Check sheet for the drawn part. Datum: minimum x, y, z corner. Units: mm. A direction names the side the tool comes from. Coordinates: 2 decimals unless noted, no trailing zeros. Write each loop counter-clockwise with the first axis right and the second up, starting at its lowest first coordinate (ties: lowest second). Pieces come first, ordered by that corner, then holes. Notation, with made-up numbers: (-9, -23.75) -> (12, -23.75) arc R24 cw to (12, -0.75) -> close; hole circle Ø4 at (37.5, -34). An arc over 180 degrees is marked (long way). One line per question, with ' | ' between items.
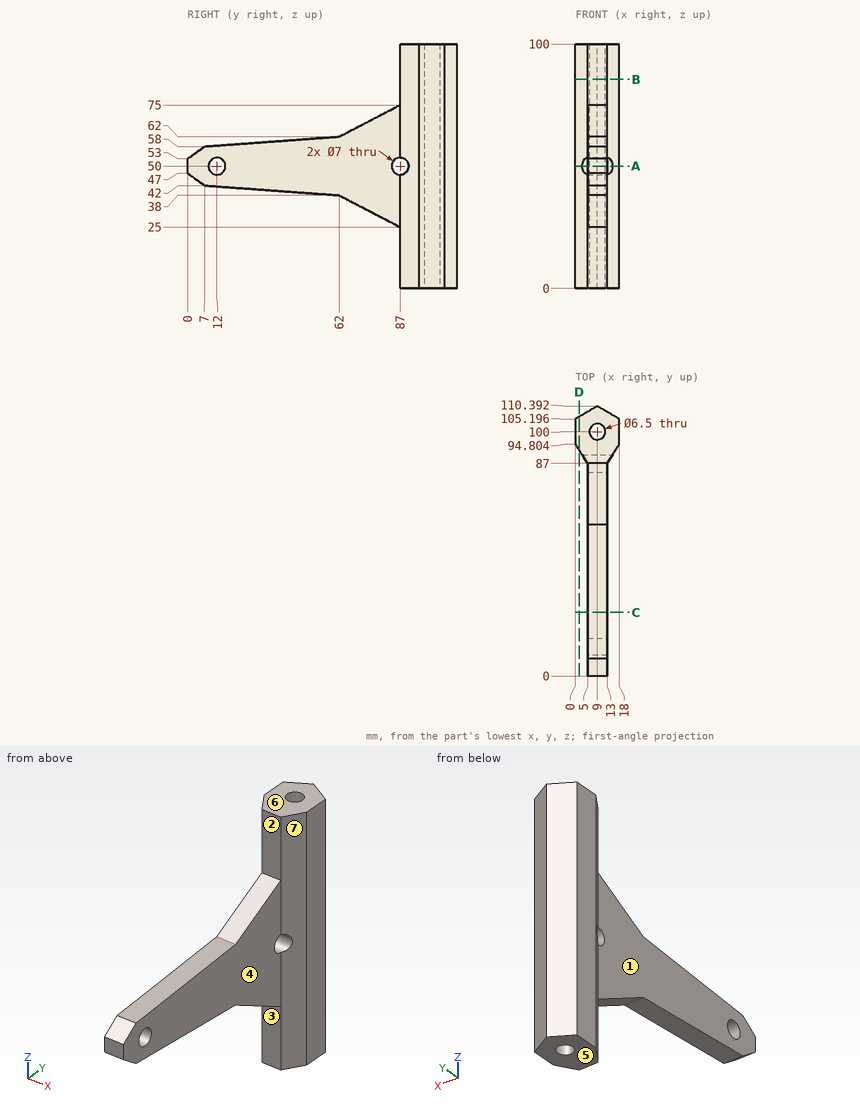
1. Tool access check on the marked faces 1, 2, 3 and 4. Record the directions out of +Z, -Z, +X, -X, +Y, -Y that give a thin tool (end or side, any length) a straight path to the whole face; none if there is none.
Worked answers:
face 1: +Z, -Z, -X, -Y | face 2: +Z, +X, -X, -Y | face 3: -Z, +X, -X, -Y | face 4: +Z, -Z, +X, -Y
2. Cross-section at C-C on y = 26. Record the boundary of the cut face in (x, z).
Worked answers:
outline: (5, 40.62) -> (13, 40.62) -> (13, 59.38) -> (5, 59.38) -> close
3. Cross-section at D-D on x = 1.5. Record the boundary of the cut face in (y, z).
Worked answers:
outline: (92.46, 0) -> (106.06, 0) -> (106.06, 100) -> (92.46, 100) -> close
4. Cross-section at A-A on z = 50. Record the boundary of the cut face in (x, y).
Worked answers:
outline: (0, 94.8) -> (2.76, 90.5) -> (15.24, 90.5) -> (18, 94.8) -> (18, 105.2) -> (9, 110.39) -> (0, 105.2) -> close; (5, 0) -> (13, 0) -> (13, 8.5) -> (5, 8.5) -> close; (5, 15.5) -> (13, 15.5) -> (13, 83.5) -> (5, 83.5) -> close; hole circle Ø6.5 at (9, 100)
5. Material ranges on line 1 (Y direction, x = 8.25, z = 50); line 2 (Y direction, x = 8, z = 50) (1 decimal); line 3 (Y direction, x = 8, z = 79) (1 decimal), recorded low to high. Write a range as from..to.
Worked answers:
line 1: 0..8.5, 15.5..83.5, 90.5..96.84, 103.16..109.96 | line 2: 0..8.5, 15.5..83.5, 90.5..96.9, 103.1..109.8 | line 3: 87..96.9, 103.1..109.8
6. Go/stop test with flat-tipped pins: P1, Ø5.5, axis at y = 12, z = 50, coming from the +X side; P2, Ø9, axis at y = 87, z = 50, coming from the +X side; P3, Ø2, axis at x = 3, z = 24, coming from the -Y side; P4, Ø2.5, axis at x = 9, z = 93.5, coming from the -Y side. Record where each tip stops, or that it passes through.
Worked answers:
P1: through | P2: x = 15.88 | P3: y = 88.56 | P4: y = 87
7. Mould release check, pull along Z, two halves, no side actions. Record for the marked faces 5, 6 and 7: released by +Z, released by -Z, zero draft, split by the parting line, or undercut.
Worked answers:
face 5: released by -Z | face 6: released by +Z | face 7: zero draft
8. Cross-section at B-B on z = 85.5. Record the boundary of the cut face in (x, y).
Worked answers:
outline: (0, 94.8) -> (5, 87) -> (13, 87) -> (18, 94.8) -> (18, 105.2) -> (9, 110.39) -> (0, 105.2) -> close; hole circle Ø6.5 at (9, 100)
